The listing builds one solid part. Answer for the finished solid, in the listing's coordinates (mm). Round coordinates to 2 decimals unless told otherwise and drop trailing zeros. Write each loop counter-clockwise with the first axis right and the second up, starting at its lowest first coordinate (ties: lowest second). Pieces come first, ordered by that corner, then holes. Notation, with made-up numbers: M -36,13.5 L 13,13.5 A18 cw 13,25.5 Z; hole C -9,-38 d8. An arc over 180 degrees is marked long. One line per item, written item: value. Start each with the question number.
(1) Section D-D (z = -15) is taken. Determine the outline of the cut face in (x, y).
(2) Section B-B (z = -2) is taken. Determine the outline of the cut face in (x, y).
(3) Section C-C (y = 0.3) is taken. Determine the outline of the cut face in (x, z), plus the area to 3 significant figures.
(4) Section A-A (x = -36) is taken. Determine the outline of the cut face in (y, z), plus the area to 3 significant figures.
(5) Consider probe 1 along X at (y, z) = (0.95, 6); probe 2 along Z at (x, y) = (34, 0.25); probe 3 along Z at (x, y) = (7, 0.8). Determine where each line is inside the solid, lowest interval first.
Autodesk Inventor part; units mm, degrees
ref_plane "YZ Plane" through (0, 0, 0) normal (1, 0, 0) x (0, 1, 0)
ref_plane "XZ Plane" through (0, 0, 0) normal (0, 1, 0) x (-1, 0, 0)
ref_plane "XY Plane" through (0, 0, 0) normal (0, 0, 1) x (1, 0, 0)
sketch "Szkic1" plane through (0, 0, 0) normal (0, 1, 0) x (-1, 0, 0)
  line L0 (-28, -40.5) -> (28, -40.5)
  line L1 (28, -40.5) -> (28, 40.5)
  line L2 (28, 40.5) -> (-28, 40.5)
  line L3 (-28, 40.5) -> (-28, -40.5)
  point P0 (0, 0)
  dimension "d0" = 81
  dimension "d1" = 56
  dimension "d2" = 28
  dimension "d3" = 40.5
extrude "Wyciągnięcie proste1" add sketch "Szkic1" along normal blind 1
sketch "Szkic2" plane through (0, 1, 0) normal (0, 1, 0) x (1, 0, 0)
  line L0 (-25.5, 9) -> (25.5, 9)
  line L1 (25.5, 9) -> (25.5, -9)
  line L2 (25.5, -9) -> (-25.5, -9)
  line L3 (-25.5, -9) -> (-25.5, 9)
  point P0 (0, 0)
  dimension "d6" = 18
  dimension "d7" = 9
  dimension "d8" = 51
  dimension "d9" = 25.5
extrude "Wyciągnięcie proste2" cut sketch "Szkic2" against normal blind 1
sketch "Szkic3" plane through (0, 1, 0) normal (0, 1, 0) x (1, 0, 0)
  line L0 (-48.5, -34.5) -> (48.5, -34.5)
  line L1 (48.5, -34.5) -> (48.5, -40.5)
  line L2 (48.5, -40.5) -> (-48.5, -40.5)
  line L3 (-48.5, -40.5) -> (-48.5, -34.5)
  line L4 (-28, -40.5) -> (28, -40.5)
  line L5 (25.5, -9) -> (-25.5, -9)
  line L6 (-48.5, 40.5) -> (48.5, 40.5)
  line L7 (48.5, 40.5) -> (48.5, 34.5)
  line L8 (48.5, 34.5) -> (-48.5, 34.5)
  line L9 (-48.5, 34.5) -> (-48.5, 40.5)
  line L10 (28, 40.5) -> (-28, 40.5)
  point P0 (0, 0)
  point P1 (28, -9.365)
  point P2 (-28, -9.365)
  point P3 (-25.5, -9)
  dimension "d12" = 97
  dimension "d13" = 6
  dimension "d15" = 48.5
  dimension "d17" = 0
  dimension "d20" = 6
  dimension "d21" = 0
  dimension "d22" = 97
  dimension "d23" = 0
extrude "Wyciągnięcie proste4" add sketch "Szkic3" against normal blind 1
properties part number "pcb_bottom"
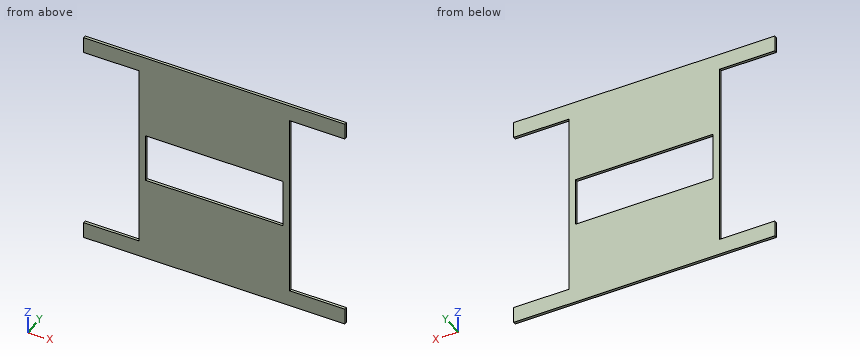
Recorded:
1. outline: M -28,0 L 28,0 L 28,1 L -28,1 Z
2. outline: M -28,0 L -25.5,0 L -25.5,1 L -28,1 Z; M 25.5,0 L 28,0 L 28,1 L 25.5,1 Z
3. outline: M -48.5,-40.5 L 48.5,-40.5 L 48.5,-34.5 L 28,-34.5 L 28,34.5 L 48.5,34.5 L 48.5,40.5 L -48.5,40.5 L -48.5,34.5 L -28,34.5 L -28,-34.5 L -48.5,-34.5 Z; hole M -25.5,-9 L 25.5,-9 L 25.5,9 L -25.5,9 Z
3. area: 4,110 mm2
4. outline: M 0,-40.5 L 1,-40.5 L 1,-34.5 L 0,-34.5 Z; M 0,34.5 L 1,34.5 L 1,40.5 L 0,40.5 Z
4. area: 12.0 mm2
5. probe 1: x = -28 to -25.5, 25.5 to 28
5. probe 2: z = -40.5 to -34.5, 34.5 to 40.5
5. probe 3: z = -40.5 to -9, 9 to 40.5
